Design review of the part shown in the three views and the two pictorial views. Dimensions are in mm from the part's minimum x, y and z. Coordinates: 2 decimals unless noted, no trailing zeros. Loops run counter-clockwise (first coordinate to the right, second up) from the corner with the lowest first, then second, coordinate; pieces in that order, holes last. Notation, with made-up numbers: (-7, -29) -> (16, -29) arc R8 ccw to (16, -22) -> close; hole circle Ø11 at (30, 65). An arc over 180 degrees is marked (long way). One line per item, written item: value.
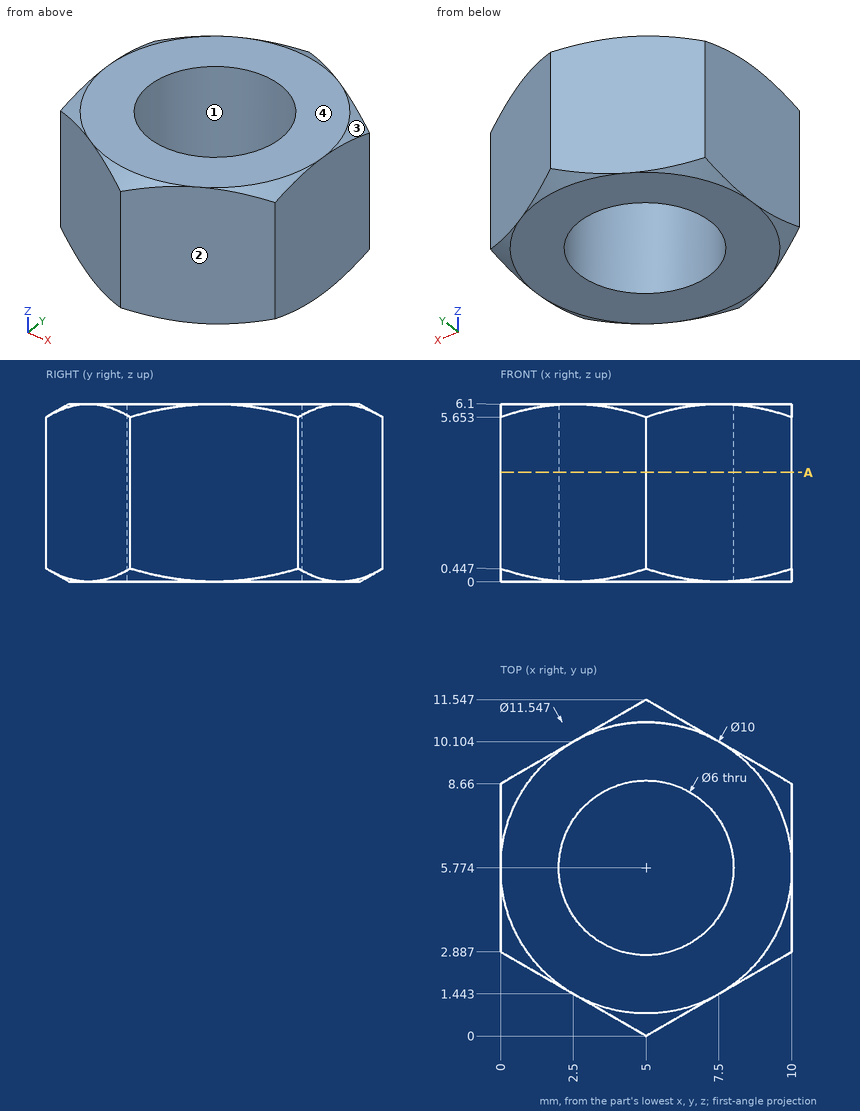
1. Take a section at A-A, the plane z = 3.75. Give the boundary of the cut face in (x, y).
Return value:
outline: (0, 2.89) -> (5, 0) -> (10, 2.89) -> (10, 8.66) -> (5, 11.55) -> (0, 8.66) -> close; hole circle Ø6 at (5, 5.77)
2. To check wall thickness, follow probe 1 along Y at (x, z) = (2.25, 2.5) (1 decimal); probe 2 along Y at (x, z) = (4.5, 4) (1 decimal); probe 3 along X at (y, z) = (4, 2.75). State the ranges of each line that lie inside material, in increasing order. Write a range as from..to.
Return value:
probe 1: y = 1.6..4.6, 7..10
probe 2: y = 0.3..2.8, 8.7..11.3
probe 3: x = 0..2.58, 7.42..10
3. Insertion check: pin 1 Ø3 at (x, y) = (4.5, 3) entering from -Z; pin 2 Ø1.5 at (x, z) = (5.5, 4) entering from +Y. Each pin has a flat end and moves straight along its axis. Give the tip position at first contact, or say it passes through.
Return value:
pin 1: stops at z = 0
pin 2: stops at y = 11.55
4. The part is to be moulded in two halves that separate along Y. For the marked faces 1, 2, 3 and 4, say which applies: pulls with the +Y half, pulls with the -Y half, needs draft (parallel to the pull), parting line crosses it, or undercut.
Return value:
face 1: undercut
face 2: pulls with the -Y half
face 3: pulls with the +Y half
face 4: needs draft
